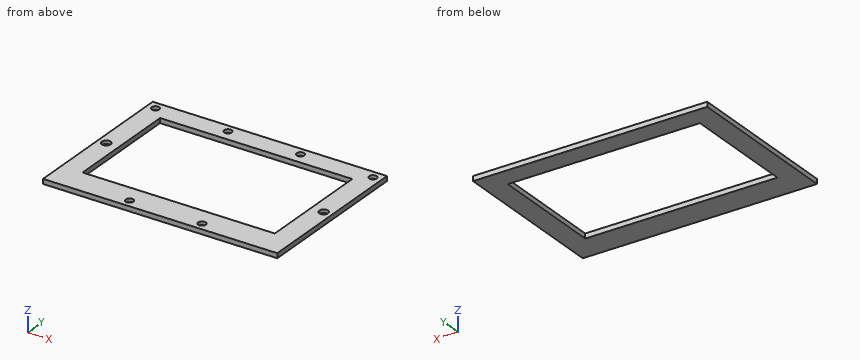
from build123d import *

# Parameters (mm, degrees)
SKETCH1_W           = 195
SKETCH1_H           = 136
SKETCH1_W_2         = 171
SKETCH1_H_2         = 112
SKETCH1_W_3         = 160
SKETCH1_H_3         = 96
SKETCH1_W_4         = 29
SKETCH1_H_4         = 3
BOSS_EXTRUDE1_DEPTH = 2
SKETCH1_3_W         = 195
SKETCH1_3_H         = 136
SKETCH1_3_W_2       = 171
SKETCH1_3_H_2       = 112
SKETCH1_3_W_3       = 160
SKETCH1_3_H_3       = 96
SKETCH1_3_W_4       = 29
SKETCH1_3_H_4       = 3
BOSS_EXTRUDE2_DEPTH = 2
SKETCH2_R           = 3.175
SKETCH2_R_2         = 3.673722566
CUT_EXTRUDE1_DEPTH  = 2.794


with BuildPart() as part:
    # Sketch1 → Boss-Extrude1 (new body)
    # profile 1 of 3: a face of its own
    with BuildSketch(Plane.XY):
        Rectangle(SKETCH1_W, SKETCH1_H)
        Polygon((85.5, 56), (85.5, -56), (14.5, -56), (14.5, -59), (-14.5, -59), (-14.5, -56), (-85.5, -56), (-85.5, 56), align=None, mode=Mode.SUBTRACT)
    # profile 2 of 3: a face of its own
    with BuildSketch(Plane.XY):
        Rectangle(SKETCH1_W_2, SKETCH1_H_2)
        with Locations((0, 3)):
            Rectangle(SKETCH1_W_3, SKETCH1_H_3, mode=Mode.SUBTRACT)
    # profile 3 of 3: a face of its own
    with BuildSketch(Plane.XY):
        with Locations((0, -57.5)):
            Rectangle(SKETCH1_W_4, SKETCH1_H_4)
    extrude(amount=-BOSS_EXTRUDE1_DEPTH)

    # Sketch1_3 → Boss-Extrude2 (add)
    # profile 1 of 3: a face of its own
    with BuildSketch(Plane.XY):
        Rectangle(SKETCH1_3_W, SKETCH1_3_H)
        Polygon((85.5, 56), (85.5, -56), (14.5, -56), (14.5, -59), (-14.5, -59), (-14.5, -56), (-85.5, -56), (-85.5, 56), align=None, mode=Mode.SUBTRACT)
    # profile 2 of 3: a face of its own
    with BuildSketch(Plane.XY):
        Rectangle(SKETCH1_3_W_2, SKETCH1_3_H_2)
        with Locations((0, 3)):
            Rectangle(SKETCH1_3_W_3, SKETCH1_3_H_3, mode=Mode.SUBTRACT)
    # profile 3 of 3: a face of its own
    with BuildSketch(Plane.XY):
        with Locations((0, -57.5)):
            Rectangle(SKETCH1_3_W_4, SKETCH1_3_H_4)
    extrude(amount=BOSS_EXTRUDE2_DEPTH)

    # Sketch2 → Cut-Extrude1 (cut)
    with BuildSketch(Plane.XY.offset(2)):
        with Locations((-90.5, 61)):
            Circle(SKETCH2_R)
        with Locations((90.5, 61)):
            Circle(SKETCH2_R)
        with Locations((-30.166666667, -61)):
            Circle(SKETCH2_R)
        with Locations((30.166666667, -61)):
            Circle(SKETCH2_R)
        with Locations((90.5, 0)):
            Circle(SKETCH2_R_2)
        with Locations((-30.166666667, 61)):
            Circle(SKETCH2_R)
        with Locations((30.166666667, 61)):
            Circle(SKETCH2_R)
        with Locations((-90.5, 0)):
            Circle(SKETCH2_R_2)
    extrude(amount=-CUT_EXTRUDE1_DEPTH, mode=Mode.SUBTRACT)


solid = part.part
Verification items for the finished model (mm, model axes). Give positions to 0.01 mm unless a question says otherwise; leave off trailing zeros. Order: outer loops, then holes, each group sorted by start corner. A loop starts at its lowest first (then second) coordinate and runs counter-clockwise, first axis right, second up. Notation, with made-up numbers: (-22, 56.25) -> (13, 56.25) arc R36 ccw to (13, 91.25) -> close; hole circle Ø8 at (21.5, -31.5). An arc over 180 degrees is marked (long way). Answer as CSV lines item,"result".
Q1. Scan lines: probe 1 along Y at (x, z) = (-30, 0.7); probe 2 along Y at (x, z) = (90.5, 1.4) (3 decimals); probe 3 along Y at (x, z) = (24, 0.6). Record each from-to range of solid material in increasing order.
Solutions:
probe 1,"y = -68 to -64.17, -57.83 to -45, 51 to 57.83, 64.17 to 68"
probe 2,"y = -68 to -3.674, 3.674 to 57.825, 64.175 to 68"
probe 3,"y = -68 to -45, 51 to 68"
Q2. Depth check by flat-ended pin: pin 1 (4 mm diameter, centred on x = -30.17, y = 61, fed in from +Z). Enter the tip coordinate at first touch or a pass-through.
Solutions:
pin 1,"stops at z = -0.79"
Q3. Sectioned sample at B-B on y = -8. Record the cut outline in (x, z), plus the area to 3 significant figures.
Solutions:
outline,"(-97.5, -2) -> (-80, -2) -> (-80, 2) -> (-97.5, 2) -> close; (80, -2) -> (97.5, -2) -> (97.5, 2) -> (80, 2) -> close"
area,"140 mm²"
Q4. Sectioned sample at C-C on z = 0.3. Count the separate pieces of the cut face and the enclosed holes in it, plus the area to 3 significant figures.
Solutions:
separate pieces,"1"
enclosed holes,"9"
area,"10,900 mm²"
Q5. Sectioned sample at D-D on x = 90.5. Record the cut outline in (y, z) (3 decimals).
Solutions:
outline,"(-68, -2) -> (68, -2) -> (68, 2) -> (64.175, 2) -> (64.175, -0.794) -> (57.825, -0.794) -> (57.825, 2) -> (3.674, 2) -> (3.674, -0.794) -> (-3.674, -0.794) -> (-3.674, 2) -> (-68, 2) -> close"
Q6. Sectioned sample at A-A on x = 22. Record the cut outline in (y, z), plus the area to 3 significant figures.
Solutions:
outline,"(-68, -2) -> (-45, -2) -> (-45, 2) -> (-68, 2) -> close; (51, -2) -> (68, -2) -> (68, 2) -> (51, 2) -> close"
area,"160 mm²"
